from build123d import *

# Parameters (mm, degrees)
ESQUISSE1_W             = 40
ESQUISSE1_H             = 30
BOSS_EXTRU_1_DEPTH      = 70
ESQUISSE2_W             = 30
ESQUISSE2_H             = 10.2
ENL_V_MAT_EXTRU_1_DEPTH = 100
CONG_1_R                = 2
ENL_V_MAT_EXTRU_2_REACH = 88.023
ENL_V_MAT_EXTRU_3_DEPTH = 5
TROU_TARAUD_M41_D       = 3.3


with BuildPart() as part:
    # Esquisse1 → Boss.-Extru.1 (new, symmetric)
    with BuildSketch(Plane(origin=(0, 0, 0), x_dir=(0, 0, -1), z_dir=(1, 0, 0))):
        with Locations((-20, 0)):
            Rectangle(ESQUISSE1_W, ESQUISSE1_H)
    extrude(amount=BOSS_EXTRU_1_DEPTH, both=True)

    # Esquisse2 → Enlèv. mat.-Extru.1 (cut, symmetric)
    with BuildSketch(Plane(origin=(0, 0, 0), x_dir=(0, 0, -1), z_dir=(1, 0, 0))):
        with Locations((-15, -0.1)):
            Rectangle(ESQUISSE2_W, ESQUISSE2_H)
    extrude(amount=ENL_V_MAT_EXTRU_1_DEPTH, both=True, mode=Mode.SUBTRACT)

    # Congé1
    cong_1_edges = [part.edges().sort_by_distance(p)[0] for p in [
        (0, 5, 0),
        (0, -5.2, 0),
        (0, -15, 0),
        (0, -15, 40),
        (0, 15, 40),
        (0, 15, 0),
    ]]
    fillet(cong_1_edges, radius=CONG_1_R)

    # Esquisse5 → Enlèv. mat.-Extru.2 (cut, up to next)
    with BuildSketch(Plane(origin=(0, 15, 0), x_dir=(1, 0, 0), z_dir=(0, 1, 0)), mode=Mode.PRIVATE) as enl_v_mat_extru_2_sk1:
        with BuildLine():
            Line((-32.25, -6), (-32.25, -26))
            ThreePointArc((-32.25, -26), (-30, -28.25), (-27.75, -26))
            Line((-27.75, -26), (-27.75, -6))
            ThreePointArc((-27.75, -6), (-30, -3.75), (-32.25, -6))
        make_face()
    enl_v_mat_extru_2_tool1 = extrude(enl_v_mat_extru_2_sk1.sketch, amount=-ENL_V_MAT_EXTRU_2_REACH, mode=Mode.PRIVATE) & part.part
    # Esquisse5 → Enlèv. mat.-Extru.2 (cut, up to next)
    with BuildSketch(Plane(origin=(0, 15, 0), x_dir=(1, 0, 0), z_dir=(0, 1, 0)), mode=Mode.PRIVATE) as enl_v_mat_extru_2_sk2:
        with BuildLine():
            Line((32.25, -6), (32.25, -26))
            ThreePointArc((32.25, -26), (30, -28.25), (27.75, -26))
            Line((27.75, -26), (27.75, -6))
            ThreePointArc((27.75, -6), (30, -3.75), (32.25, -6))
        make_face()
    enl_v_mat_extru_2_tool2 = extrude(enl_v_mat_extru_2_sk2.sketch, amount=-ENL_V_MAT_EXTRU_2_REACH, mode=Mode.PRIVATE) & part.part
    add(enl_v_mat_extru_2_tool1.solids().sort_by_distance((-30, 15, 16))[0], mode=Mode.SUBTRACT)
    add(enl_v_mat_extru_2_tool2.solids().sort_by_distance((30, 15, 16))[0], mode=Mode.SUBTRACT)

    # Esquisse6 → Enlèv. mat.-Extru.3 (cut)
    with BuildSketch(Plane(origin=(0, 15, 0), x_dir=(1, 0, 0), z_dir=(0, 1, 0))):
        with BuildLine():
            Line((-34, -6), (-34, -26))
            ThreePointArc((-34, -26), (-30, -30), (-26, -26))
            Line((-26, -26), (-26, -6))
            ThreePointArc((-26, -6), (-30, -2), (-34, -6))
        make_face()
        with BuildLine():
            Line((26, -6), (26, -26))
            ThreePointArc((26, -26), (30, -30), (34, -26))
            Line((34, -26), (34, -6))
            ThreePointArc((34, -6), (30, -2), (26, -6))
        make_face()
    extrude(amount=-ENL_V_MAT_EXTRU_3_DEPTH, mode=Mode.SUBTRACT)

    # Trou taraudé M41 (through all)
    with Locations(Plane.XY.offset(40)):
        with Locations((-30, 0), (30, 0)):
            Hole(TROU_TARAUD_M41_D / 2)


solid = part.part
Input: part model. Units: mm. Frame: model coordinates. A direction names the side the tool comes from. Give positions to 0.01 mm unless a question says otherwise; leave off trailing zeros. Order: outer loops, then holes, each group sorted by start corner. A loop starts at its lowest first (then second) coordinate and runs counter-clockwise, first axis right, second up. Notation, with made-up numbers: (-6, 41) - (22, 41) arc R24 ccw to (22, 76) - close; hole circle Ø6 at (-37, 3). An arc over 180 degrees is marked (long way). Answer as a JSON object with one key per item and string values. Group by question number.
Q1. First-contact query: pin 1 Ø6.5 at (x, z) = (-30.5, 9) entering from +Y; pin 2 Ø5 at (x, y) = (22.5, -2) entering from -Z. Flat tips, straight axial feed; report the tip coordinate or a pass-through.
Q2. Mould query, pull axis Z, two halves, no side actions, for faces 1 (the face through (-28.35, 0.07, 34.93)), 2 (the face through (30, 13, 30)). Classes: pulls with the +Z half, pulls with the -Z half, needs draft (parallel to the pull), parting line crosses it, or undercut.
Q3. Cut plane C-C, the plane x = -45. Output: boundary loops of the cut face in (y, z).
Q4. Cut plane B-B, the plane z = 23. Output: boundary loops of the cut face in (x, y), then the cut area to 3 significant figures.
Q5. Set-up query: faces 3 (the face through (1, -15, 20)), 4 (the face through (1, 5, 16)), 5 (the face through (26, 13, 16)). Return all of +Z, -Z, +X, -X, +Y, -Y with unobstructed straight access to the full face (end or side cutting, diameter ignored); none if empty.
Q6. Line query: probe 1 along X at (y, z) = (12.5, 12); probe 2 along X at (y, z) = (-1.5, 32.5); probe 3 along Y at (x, z) = (30, 33.5). Output: solid intervals per line, ascending.
Q7. Cut plane A-A, the plane y = 0. Output: boundary loops of the cut face in (x, z).
Results:
{
 "1": {"pin 1": "y = 10", "pin 2": "z = 30"},
 "2": {"face 1": "needs draft", "face 2": "undercut"},
 "3": {"outline": "(-15, 2) arc R2 ccw to (-13, 0) - (-7.2, 0) arc R2 ccw to (-5.2, 2) - (-5.2, 30) - (5, 30) - (5, 2) arc R2 ccw to (7, 0) - (13, 0) arc R2 ccw to (15, 2) - (15, 38) arc R2 ccw to (13, 40) - (-13, 40) arc R2 ccw to (-15, 38) - close"},
 "4": {"outline": "(-70, -15) - (70, -15) - (70, -5.2) - (-70, -5.2) - close; (-70, 5) - (-32.25, 5) - (-32.25, 10) - (-34, 10) - (-34, 15) - (-70, 15) - close; (-27.75, 5) - (27.75, 5) - (27.75, 10) - (26, 10) - (26, 15) - (-26, 15) - (-26, 10) - (-27.75, 10) - close; (32.25, 5) - (70, 5) - (70, 15) - (34, 15) - (34, 10) - (32.25, 10) - close", "area": "2,650 mm^2"},
 "5": {"face 3": "+Z, -Z, +X, -X, -Y", "face 4": "-Z, +X, -X", "face 5": "+Y"},
 "6": {"probe 1": "-70 to -34, -26 to 26, 34 to 70", "probe 2": "-70 to -30.69, -29.31 to 29.31, 30.69 to 70", "probe 3": "-15 to -1.65, 1.65 to 15"},
 "7": {"outline": "(-70, 30) - (-31.65, 30) - (-31.65, 40) - (-70, 40) - close; (-28.35, 30) - (28.35, 30) - (28.35, 40) - (-28.35, 40) - close; (31.65, 30) - (70, 30) - (70, 40) - (31.65, 40) - close"}
}
